from build123d import *

# Parameters (mm, degrees)
F1_DEPTH = 25
F2_W     = 15.5
F2_H     = 10
F3_DEPTH = 30.2


with BuildPart() as f1:
    # F0 (on Front) → F1 (new body)
    with BuildSketch(Plane.XZ):
        Polygon((20.2, 0), (0, 0), (0, 15), (-5, 15), (-5, -15), (25.2, -15), (25.2, 15), (20.2, 15), align=None)
    extrude(amount=F1_DEPTH)

    # F2 (on face) → F3 (cut, through all)
    with BuildSketch(Plane.YZ.offset(25.2)):
        with Locations((-12.5, -10)):
            Rectangle(F2_W, F2_H)
    extrude(amount=-F3_DEPTH, mode=Mode.SUBTRACT)


solid = f1.part
For this review, take the finished solid that the model builds, in its own axes (mm). A direction names the side the tool comes from. Give positions to 0.01 mm unless a question says otherwise; leave off trailing zeros. Loops run counter-clockwise (first coordinate to the right, second up) from the corner with the lowest first, then second, coordinate; pieces in that order, holes last. Notation, with made-up numbers: M 52,4 L 76,4 A13 cw 76,11 Z; hole C 23,-20.5 d5. An arc over 180 degrees is marked long. Put each result on its own line as item: value. Start each with the question number.
(1) Add section B-B, the plane y = -7. Write out the cut boundary in (x, z).
(2) Machinability: for faces 1 (the flat face through (10, -20.25, -10)), 2 (the flat face through (0, -12, 7)), 3 (the flat face through (10, 0, -3)), which of the approach directions +Z, -Z, +X, -X, +Y, -Y give a long, thin tool a straight path to every point of the face, cutting with its end or side? Answer none if there is none.
(3) For pin 1 (12 mm diameter, centred on x = 5, z = 1.5, fed in from -Y); pin 2 (8 mm diameter, centred on x = 12.5, y = -14.5, fed in from -Z), all flat-tipped, find the tip position at first contact; note any pin that passes through.
(4) Add section D-D, the plane z = 8.25. Write out the cut boundary in (x, y), then the cut area to 3 significant figures.
(5) Add section A-A, the plane z = -10. Write out the cut boundary in (x, y), then the cut area to 3 significant figures.
(6) Wall thickness on L1, parallel to Y at x = 16.5, z = -9.75; L2, parallel to X at y = -3.5, z = 3.5; L3, parallel to Z at x = 8, y = -2.25: over which ranges is each line inside the solid? List them lowest first.
(7) The part is to be moulded in two halves that separate along X. For faces 4 (the flat face through (10, -13, -5)), 5 (the flat face through (10, -12, 0)), 6 (the flat face through (25.2, -12, 3)), say which applies: +X half, -X half, draft (parallel to the pull), parting line (faces both ways), or undercut.
(8) Add section C-C, the plane x = 15.5. Write out the cut boundary in (y, z).
Result:
1. outline: M -5,-5 L 25.2,-5 L 25.2,15 L 20.2,15 L 20.2,0 L 0,0 L 0,15 L -5,15 Z
2. face 1: -Z, +X, -X
2. face 2: +Z, +Y, -Y
2. face 3: +Z, -Z, +X, -X, +Y
3. pin 1: stops at y = -25
3. pin 2: stops at z = -5
4. outline: M -5,-25 L 0,-25 L 0,0 L -5,0 Z; M 20.2,-25 L 25.2,-25 L 25.2,0 L 20.2,0 Z
4. area: 250 mm^2
5. outline: M -5,-25 L 25.2,-25 L 25.2,-20.25 L -5,-20.25 Z; M -5,-4.75 L 25.2,-4.75 L 25.2,0 L -5,0 Z
5. area: 287 mm^2
6. L1: y = -25 to -20.25, -4.75 to 0
6. L2: x = -5 to 0, 20.2 to 25.2
6. L3: z = -15 to 0
7. face 4: draft
7. face 5: undercut
7. face 6: +X half
8. outline: M -25,-15 L -20.25,-15 L -20.25,-5 L -4.75,-5 L -4.75,-15 L 0,-15 L 0,0 L -25,0 Z
